```python
from build123d import *

# Parameters (mm, degrees)
SKETCH4_R           = 38.1
BOSS_EXTRUDE3_DEPTH = 5
SKETCH5_R           = 18.9
BOSS_EXTRUDE4_DEPTH = 33
FILLET4_R           = 3
CUT_EXTRUDE4_DEPTH  = 39.48


with BuildPart() as part:
    # Sketch4 → Boss-Extrude3 (new body)
    with BuildSketch(Plane.XY):
        Circle(SKETCH4_R)
        with BuildLine():
            Line((-68.1, 0), (-38.1, 0))
            ThreePointArc((-38.1, 0), (-38.017533534, 2.505422923), (-37.770491127, 5))
            Line((-37.770491127, 5), (-68.1, 5))
            Line((-68.1, 5), (-68.1, 0))
        make_face()
        with BuildLine():
            ThreePointArc((-37.770491127, -5), (-38.017533534, -2.505422923), (-38.1, 0))
            Line((-38.1, 0), (-68.1, 0))
            Line((-68.1, 0), (-68.1, -5))
            Line((-68.1, -5), (-37.770491127, -5))
        make_face()
        with BuildLine():
            Line((-68.1, 0), (-68.1, 5))
            ThreePointArc((-68.1, 5), (-73.1, 0), (-68.1, -5))
            Line((-68.1, -5), (-68.1, 0))
        make_face()
    extrude(amount=BOSS_EXTRUDE3_DEPTH)

    # Sketch5 → Boss-Extrude4 (add)
    with BuildSketch(Plane.XY.offset(5)):
        Circle(SKETCH5_R)
    extrude(amount=BOSS_EXTRUDE4_DEPTH)

    # Fillet4
    fillet4_edges = [part.edges().sort_by_distance(p)[0] for p in [
        (-18.9, 0, 5),
    ]]
    fillet(fillet4_edges, radius=FILLET4_R)

    # Sketch6 → Cut-Extrude4 (cut)
    with BuildSketch(Plane.XY.offset(38)):
        with BuildLine():
            Line((2.38156986, 12.481406461), (0, 13.856406461))
            Line((0, 13.856406461), (-2.38156986, 12.481406461))
            ThreePointArc((-2.38156986, 12.481406461), (0, 11.106406461), (2.38156986, 12.481406461))
        make_face()
        with BuildLine():
            Line((-2.38156986, 12.481406461), (0, 13.856406461))
            Line((0, 13.856406461), (2.38156986, 12.481406461))
            ThreePointArc((2.38156986, 12.481406461), (2.656296022, 13.144654087), (2.75, 13.856406461))
            ThreePointArc((2.75, 13.856406461), (-0.711752374, 16.512702483), (-2.38156986, 12.481406461))
        make_face()
        with BuildLine():
            ThreePointArc((14.75, 6.92820323), (12.711752374, 9.584499253), (9.61843014, 8.30320323))
            Line((9.61843014, 8.30320323), (12, 6.92820323))
            Line((12, 6.92820323), (12, 4.17820323))
            ThreePointArc((12, 4.17820323), (13.944543648, 4.983659582), (14.75, 6.92820323))
        make_face()
        with BuildLine():
            Line((12, 6.92820323), (9.61843014, 8.30320323))
            ThreePointArc((9.61843014, 8.30320323), (9.61843014, 5.55320323), (12, 4.17820323))
            Line((12, 4.17820323), (12, 6.92820323))
        make_face()
        with BuildLine():
            ThreePointArc((14.75, -6.92820323), (13.944543648, -4.983659582), (12, -4.17820323))
            Line((12, -4.17820323), (12, -6.92820323))
            Line((12, -6.92820323), (9.61843014, -8.30320323))
            ThreePointArc((9.61843014, -8.30320323), (12.711752374, -9.584499253), (14.75, -6.92820323))
        make_face()
        with BuildLine():
            Line((12, -6.92820323), (12, -4.17820323))
            ThreePointArc((12, -4.17820323), (9.61843014, -5.55320323), (9.61843014, -8.30320323))
            Line((9.61843014, -8.30320323), (12, -6.92820323))
        make_face()
        with BuildLine():
            ThreePointArc((-9.25, 6.92820323), (-9.343703978, 7.639955604), (-9.61843014, 8.30320323))
            Line((-9.61843014, 8.30320323), (-12, 6.92820323))
            Line((-12, 6.92820323), (-12, 4.17820323))
            ThreePointArc((-12, 4.17820323), (-10.055456352, 4.983659582), (-9.25, 6.92820323))
        make_face()
        with BuildLine():
            Line((-12, 6.92820323), (-9.61843014, 8.30320323))
            ThreePointArc((-9.61843014, 8.30320323), (-14.38156986, 8.30320323), (-12, 4.17820323))
            Line((-12, 4.17820323), (-12, 6.92820323))
        make_face()
        with BuildLine():
            ThreePointArc((-9.25, -6.92820323), (-10.055456352, -4.983659582), (-12, -4.17820323))
            Line((-12, -4.17820323), (-12, -6.92820323))
            Line((-12, -6.92820323), (-9.61843014, -8.30320323))
            ThreePointArc((-9.61843014, -8.30320323), (-9.343703978, -7.639955604), (-9.25, -6.92820323))
        make_face()
        with BuildLine():
            Line((-12, -6.92820323), (-12, -4.17820323))
            ThreePointArc((-12, -4.17820323), (-14.38156986, -8.30320323), (-9.61843014, -8.30320323))
            Line((-9.61843014, -8.30320323), (-12, -6.92820323))
        make_face()
        with BuildLine():
            ThreePointArc((2.38156986, -12.481406461), (0, -11.106406461), (-2.38156986, -12.481406461))
            Line((-2.38156986, -12.481406461), (0, -13.856406461))
            Line((0, -13.856406461), (2.38156986, -12.481406461))
        make_face()
        with BuildLine():
            Line((0, -13.856406461), (-2.38156986, -12.481406461))
            ThreePointArc((-2.38156986, -12.481406461), (-0.711752374, -16.512702483), (2.75, -13.856406461))
            ThreePointArc((2.75, -13.856406461), (2.656296022, -13.144654087), (2.38156986, -12.481406461))
            Line((2.38156986, -12.481406461), (0, -13.856406461))
        make_face()
    extrude(amount=-CUT_EXTRUDE4_DEPTH, mode=Mode.SUBTRACT)


solid = part.part
```
Can you work these out from the model? Positions are in its coordinate system, mm. A direction names the side the tool comes from. Round coordinates to 2 decimals unless told otherwise and drop trailing zeros. Loops run counter-clockwise (first coordinate to the right, second up) from the corner with the lowest first, then second, coordinate; pieces in that order, holes last.
Item 1: Please list where these lines run through material, in increasing order: L1, parallel to Y at x = -12, z = 27; L2, parallel to Z at x = -55.5, y = 2; L3, parallel to X at y = 9, z = 27.
Item 2: Suppose I cut it at A-A, the plane x = 0. Write out the boundary of the cut face in (y, z), then the cut area to 3 significant figures.
Item 3: Which directions (+Z, -Z, +X, -X, +Y, -Y) give clear straight access to the entire face, cutting with the end or side of a thin tool? Please do faces 1 (the flat face through (-18, -16, 5)), 2 (the flat face through (-53, -5, 2)), 3 (the flat face through (-53, 5, 2)).
Item 4: Will these pins go through, and if not, where does the flat tip stop? pin 1 Ø7 at (x, y) = (0, -13.86) entering from +Z; pin 2 Ø4 at (x, z) = (-59.5, 1.5) entering from +Y; pin 3 Ø2 at (y, z) = (-9, 4) entering from +X; pin 4 Ø5.5 at (x, z) = (-58, 2) entering from -Y.
Item 5: Suppose I cut it at B-B, the plane z = 21. Write out the boundary of the cut face in (x, y).
Item 6: Suppose I cut it at C-C, the plane y = 0. Write out the boundary of the cut face in (x, z).
Item 7: Suppose I cut it at D-D, the plane x = -49. Write out the boundary of the cut face in (y, z), then the cut area to 3 significant figures.
Reported:
1. L1: y = -14.6 to -9.68, -4.18 to 4.18, 9.68 to 14.6
1. L2: z = 0 to 5
1. L3: x = -16.62 to -13.81, -10.19 to 10.19, 13.81 to 16.62
2. outline: (-38.1, 0) - (-16.61, 0) - (-16.61, 38) - (-18.9, 38) - (-18.9, 8) arc R3 cw to (-21.9, 5) - (-38.1, 5) - close; (-11.11, 0) - (11.11, 0) - (11.11, 38) - (-11.11, 38) - close; (16.61, 0) - (38.1, 0) - (38.1, 5) - (21.9, 5) arc R3 cw to (18.9, 8) - (18.9, 38) - (16.61, 38) - close
2. area: 1,210 mm2
3. face 1: +Z
3. face 2: +Z, -Z, -X, -Y
3. face 3: +Z, -Z, -X, +Y
4. pin 1: stops at z = 38
4. pin 2: stops at y = 5
4. pin 3: stops at x = 37.25
4. pin 4: stops at y = -5
5. outline: circle Ø37.8 at (0, 0); hole circle Ø5.5 at (-12, -6.93); hole circle Ø5.5 at (-12, 6.93); hole circle Ø5.5 at (0, -13.86); hole circle Ø5.5 at (0, 13.86); hole circle Ø5.5 at (12, -6.93); hole circle Ø5.5 at (12, 6.93)
6. outline: (-73.1, 0) - (38.1, 0) - (38.1, 5) - (21.9, 5) arc R3 cw to (18.9, 8) - (18.9, 38) - (-18.9, 38) - (-18.9, 8) arc R3 cw to (-21.9, 5) - (-73.1, 5) - close
7. outline: (-5, 0) - (5, 0) - (5, 5) - (-5, 5) - close
7. area: 50.0 mm2
